```python
from build123d import *

# Parameters (mm, degrees)
SKETCH1_R           = 6.096
BOSS_EXTRUDE1_DEPTH = 4.445
SKETCH5_R           = 7.366
BOSS_EXTRUDE4_DEPTH = 1.27
SKETCH8_R           = 8.636
CUT_EXTRUDE4_DEPTH  = 4.445
SKETCH6_R           = 1.524
CUT_EXTRUDE2_DEPTH  = 6.715
SKETCH7_W           = 9.525
SKETCH7_H           = 4.445
CUT_EXTRUDE3_DEPTH  = 3.175


with BuildPart() as part:
    # Sketch1 → Boss-Extrude1 (new body)
    with BuildSketch(Plane(origin=(0, 0, 0), x_dir=(1, 0, 0), z_dir=(0, 1, 0))):
        with BuildLine():
            Line((-10.541, 0), (-10.541, 10.668))
            Line((-10.541, 10.668), (-20.066, 10.668))
            Line((-20.066, 10.668), (-20.066, 13.843))
            Line((-20.066, 13.843), (-7.366, 13.843))
            Line((-7.366, 13.843), (7.366, 13.843))
            Line((7.366, 13.843), (20.066, 13.843))
            Line((20.066, 13.843), (20.066, 10.668))
            Line((20.066, 10.668), (10.541, 10.668))
            Line((10.541, 10.668), (10.541, 0))
            ThreePointArc((10.541, 0), (0, -10.541), (-10.541, 0))
        make_face()
        Circle(SKETCH1_R, mode=Mode.SUBTRACT)
    extrude(amount=BOSS_EXTRUDE1_DEPTH)

    # Sketch5 → Boss-Extrude4 (add)
    with BuildSketch(Plane.XZ):
        with BuildLine():
            Line((-10.541, 0), (-10.541, -10.668))
            Line((-10.541, -10.668), (-10.541, -13.843))
            Line((-10.541, -13.843), (10.541, -13.843))
            Line((10.541, -13.843), (10.541, -10.668))
            Line((10.541, -10.668), (10.541, 0))
            ThreePointArc((10.541, 0), (0, 10.541), (-10.541, 0))
        make_face()
        Circle(SKETCH5_R, mode=Mode.SUBTRACT)
    extrude(amount=BOSS_EXTRUDE4_DEPTH)

    # Sketch8 → Cut-Extrude4 (cut)
    with BuildSketch(Plane(origin=(0, 4.445, 0), x_dir=(1, 0, 0), z_dir=(0, 1, 0))):
        Circle(SKETCH8_R)
    extrude(amount=-CUT_EXTRUDE4_DEPTH, mode=Mode.SUBTRACT)

    # Sketch6 → Cut-Extrude2 (cut, through all)
    with BuildSketch(Plane(origin=(0, 4.445, 0), x_dir=(1, 0, 0), z_dir=(0, 1, 0))):
        with Locations((4.6355, 9.9695)):
            Circle(SKETCH6_R)
        with Locations((-4.6355, 9.9695)):
            Circle(SKETCH6_R)
    extrude(amount=-CUT_EXTRUDE2_DEPTH, mode=Mode.SUBTRACT)

    # Sketch7 → Cut-Extrude3 (cut)
    with BuildSketch(Plane.XY.offset(-10.668)):
        with Locations((15.3035, 2.2225)):
            Rectangle(SKETCH7_W, SKETCH7_H)
        with Locations((-15.3035, 2.2225)):
            Rectangle(SKETCH7_W, SKETCH7_H)
    extrude(amount=-CUT_EXTRUDE3_DEPTH, mode=Mode.SUBTRACT)


solid = part.part
```
Could you check a few things on this model? Use its own coordinates, in mm. A direction names the side the tool comes from. Coordinates: 2 decimals unless noted, no trailing zeros. Order: outer loops, then holes, each group sorted by start corner. A loop starts at its lowest first (then second) coordinate and runs counter-clockwise, first axis right, second up. Notation, with made-up numbers: M -33,56.5 L 4,56.5 A17 cw 4,61.5 Z; hole C -26.75,66.5 d11. An arc over 180 degrees is marked long. Use one line per item in the form item = value. Start each with the question number.
1. Suppose I cut it at A-A on x = 0. Write out the boundary of the cut face in (y, z) (3 decimals), then the cut area to 3 significant figures.
2. We'd pull the mould along X, two halves only. Please class faces 1 (the cylindrical face through (3.399, -0.626, -6.535)), 2 (the flat face through (-10.541, 2, -7)), 3 (the flat face through (0, 4.445, -10)), 4 (the cylindrical face through (4.44, 1.63, -11.48)): +X half, -X half, draft (parallel to the pull), parting line (faces both ways), or undercut.
3. Please list where these lines run through material, in increasing order: line 1 (Z direction, x = 0, y = -0.75); line 2 (Z direction, x = 3.5, y = 3.7); line 3 (Z direction, x = -4.75, y = 0.9).
4. On a 3-axis mill with a long thin cutter (end or side, diameter ignored), from which of +Z, -Z, +X, -X, +Y, -Y can I reach the whole of each face in a straight line? I mean faces 5 (the cylindrical face through (-1.124, 2.254, -8.563)), 6 (the flat face through (10.541, 2, -7)). Say none if no direction works.
5. Suppose I cut it at C-C on y = 3.55. Write out the boundary of the cut face in (x, z).
6. Suppose I cut it at D-D on x = 8.25. Write out the boundary of the cut face in (y, z) (3 decimals).
7. Suppose I cut it at B-B on x = -5.5. Write out the boundary of the cut face in (y, z) (3 decimals).
8. For pin 1 (1.5 mm diameter, centred on x = -6, y = 3.5, fed in from +Z); pin 2 (1 mm diameter, centred on x = 1, y = 3.5, fed in from +Z), each with a flat end and sliding along its axis, tell me the tip position at first contact or that it passes through.
Geometry says:
q1.outline = M -1.27,-13.843 L 4.445,-13.843 L 4.445,-8.636 L 0,-8.636 L 0,-7.366 L -1.27,-7.366 Z; M -1.27,7.366 L 0,7.366 L 0,8.636 L 4.445,8.636 L 4.445,10.541 L -1.27,10.541 Z
q1.area = 43.9 mm^2
q2.face_1 = undercut
q2.face_2 = -X half
q2.face_3 = draft
q2.face_4 = undercut
q3.line_1 = -13.84 to -7.37, 7.37 to 10.54
q3.line_2 = -13.84 to -10.99, -8.95 to -7.89, 7.89 to 9.94
q3.line_3 = -13.84 to -11.49, -8.45 to -7.21, 7.21 to 9.41
q4.face_5 = +Y
q4.face_6 = +Z, -Z, +X, +Y, -Y
q5.outline = M -10.54,-13.84 L 10.54,-13.84 L 10.54,0 A10.54 ccw -10.54,0 Z; hole C 0,0 d17.27; hole C -4.64,-9.97 d3.05; hole C 4.64,-9.97 d3.05
q6.outline = M -1.27,-13.843 L 4.445,-13.843 L 4.445,-2.553 L 0,-2.553 L 0,2.553 L 4.445,2.553 L 4.445,6.561 L -1.27,6.561 Z
q7.outline = M -1.27,-13.843 L 4.445,-13.843 L 4.445,-11.225 L -1.27,-11.225 Z; M -1.27,-8.714 L 4.445,-8.714 L 4.445,-6.658 L 0,-6.658 L 0,-4.9 L -1.27,-4.9 Z; M -1.27,4.9 L 0,4.9 L 0,6.658 L 4.445,6.658 L 4.445,8.992 L -1.27,8.992 Z
q8.pin_1 = 9.14
q8.pin_2 = 10.53
